The model under review builds one solid part; all positions refer to its coordinate system, in mm. A direction names the side the tool comes from. Give positions to 0.01 mm unless a question says otherwise; leave off trailing zeros. Order: outer loops, then holes, each group sorted by start corner. A loop starts at its lowest first (then second) coordinate and runs counter-clockwise, first axis right, second up. Notation, with made-up numbers: (57, 22.25) - (63, 22.25) arc R32 cw to (63, 55.25) - close; hole circle Ø3 at (-24.5, 88.5). An arc over 180 degrees is marked (long way). Use a Markdown table: item, result. Add a question column.
Autodesk Inventor part; units mm, degrees
ref_plane "YZ Plane" through (0, 0, 0) normal (1, 0, 0) x (0, 1, 0)
ref_plane "XZ Plane" through (0, 0, 0) normal (0, 1, 0) x (-1, 0, 0)
ref_plane "XY Plane" through (0, 0, 0) normal (0, 0, 1) x (1, 0, 0)
sketch "Esquisse1" plane through (0, 0, 0) normal (0, 1, 0) x (-1, 0, 0)
  line L0 (-5, 50) -> (5, 50)
  line L1 (5, 50) -> (5, -50)
  line L2 (5, -50) -> (-5, -50)
  line L3 (-5, -50) -> (-5, 50)
  line L4 (-5, 50) -> (5, -50) construction
  line L5 (5, 50) -> (-5, -50) construction
  point P0 (0, 0)
  dimension "d0" = 10
  dimension "d1" = 100
extrude "Extrusion1" add sketch "Esquisse1" along normal blind 10
sketch "Esquisse2" plane through (-5, 0, -50) normal (-1, 0, 0) x (0, 0, 1)
  line L0 (0, 0) -> (100, 0)
  line L1 (100, 0) -> (100, 10)
  point P0 (50, 0)
  point P1 (5, 5)
  point P2 (95, 5)
hole "Perçage1" at (-5, 5, -45) at (-5, 5, 45) direction (1, 0, 0) diameter 5 end through all
sketch "Esquisse4" plane through (-5, 0, -50) normal (-1, 0, 0) x (0, 0, 1)
  line L0 (100, 10) -> (0, 10)
  line L1 (30, 10) -> (70, 10)
  line L2 (70, 10) -> (70, 0)
  line L3 (0, 0) -> (100, 0)
  line L4 (70, 0) -> (30, 0)
  line L5 (30, 0) -> (30, 10)
  point P0 (50, 0)
extrude "Extrusion2" add sketch "Esquisse4" along normal blind 10
mirror "Symétrie1" about plane through (0, 0, 0) normal (1, 0, 0) of "Extrusion2"
sketch "Esquisse5" plane through (0, 10, 0) normal (0, 1, 0) x (1, 0, 0)
  point P0 (0, 0)
  point P1 (0, 0)
hole "Perçage2" at (0, 10, 0) direction (0, -1, 0) diameter 9 end through all
ref_plane "Plan de construction1" through (0, 0, 0) normal (1, 0, 0) x (0, 1, 0)
properties part number "Support poulie"
Q1. Draft analysis for pull direction Z (two halves, no side actions). For faces 1 (the flat face through (-5, 5, -35)), 2 (the flat face through (-10, 5, -20)), 3 (the cylindrical face through (0.07, 5.96, -42.69)), state which applies: pulls with the +Z half, pulls with the -Z half, needs draft (parallel to the pull), parting line crosses it, or undercut.
Q2. We need section D-D (y = 1). Write out the cut boundary in (x, z), plus the area to 3 significant figures.
Q3. We need section B-B (x = 0). Write out the cut boundary in (y, z).
Q4. Wall thickness on probe 1 along Z at (x, y) = (-0.25, 5); probe 2 along Y at (x, z) = (-0.25, -45); probe 3 along Z at (x, y) = (0, 3): over which ranges is each line inside the solid? List them lowest first.
Q5. We need section C-C (z = 0). Write out the cut boundary in (x, y), plus the area to 3 significant figures.
Q6. We need section A-A (y = 5). Write out the cut boundary in (x, z), plus the area to 3 significant figures.
Q7. Machinability: for faces 4 (the flat face through (-5, 5, 35)), 5 (the flat face through (-6, 10, 1)), 6 (the flat face through (0, 5, 50)), 7 (the flat face through (5, 5, 35)), 8 (the flat face through (10, 5, -20)), which of the approach directions +Z, -Z, +X, -X, +Y, -Y give a long, thin tool a straight path to every point of the face, cutting with its end or side? Answer none if there is none.
Q8. Clearance check with flat-ended pins moving along their axes: P1, Ø4.5, axis at y = 5, z = 45, coming from the -X side; P2, Ø6, axis at y = 5, z = -45, coming from the -X side; P3, Ø3, axis at x = 10, y = 4.5, coming from the +Z side; P4, Ø6, axis at y = 3.5, z = -24, coming from the +X side. State where each tip first meets the part, or that it passes through.
Here are the results:
| question | item | result |
|---|---|---|
| 1 | face 1 | needs draft |
| 1 | face 2 | pulls with the -Z half |
| 1 | face 3 | undercut |
| 2 | outline | (-15, -20) - (-5, -20) - (-5, -50) - (5, -50) - (5, -20) - (15, -20) - (15, 20) - (5, 20) - (5, 50) - (-5, 50) - (-5, 20) - (-15, 20) - close; hole circle Ø9 at (0, 0) |
| 2 | area | 1,740 mm2 |
| 3 | outline | (0, -50) - (10, -50) - (10, -4.5) - (0, -4.5) - close; (0, 4.5) - (10, 4.5) - (10, 50) - (0, 50) - close; hole circle Ø5 at (5, -45); hole circle Ø5 at (5, 45) |
| 4 | probe 1 | -50 to -47.5, -42.5 to -4.49, 4.49 to 42.5, 47.5 to 50 |
| 4 | probe 2 | 0 to 2.5, 7.5 to 10 |
| 4 | probe 3 | -50 to -46.5, -43.5 to -4.5, 4.5 to 43.5, 46.5 to 50 |
| 5 | outline | (-15, 0) - (-4.5, 0) - (-4.5, 10) - (-15, 10) - close; (4.5, 0) - (15, 0) - (15, 10) - (4.5, 10) - close |
| 5 | area | 210 mm2 |
| 6 | outline | (-15, -20) - (-5, -20) - (-5, -42.5) - (5, -42.5) - (5, -20) - (15, -20) - (15, 20) - (5, 20) - (5, 42.5) - (-5, 42.5) - (-5, 20) - (-15, 20) - close; (-5, -50) - (5, -50) - (5, -47.5) - (-5, -47.5) - close; (-5, 47.5) - (5, 47.5) - (5, 50) - (-5, 50) - close; hole circle Ø9 at (0, 0) |
| 6 | area | 1,640 mm2 |
| 7 | face 4 | +Z, -X, +Y, -Y |
| 7 | face 5 | +Z, -Z, +X, -X, +Y |
| 7 | face 6 | +Z, +X, -X, +Y, -Y |
| 7 | face 7 | +Z, +X, +Y, -Y |
| 7 | face 8 | -Z, +X, +Y, -Y |
| 8 | P1 | through |
| 8 | P2 | x = -5 |
| 8 | P3 | z = 20 |
| 8 | P4 | x = 5 |
